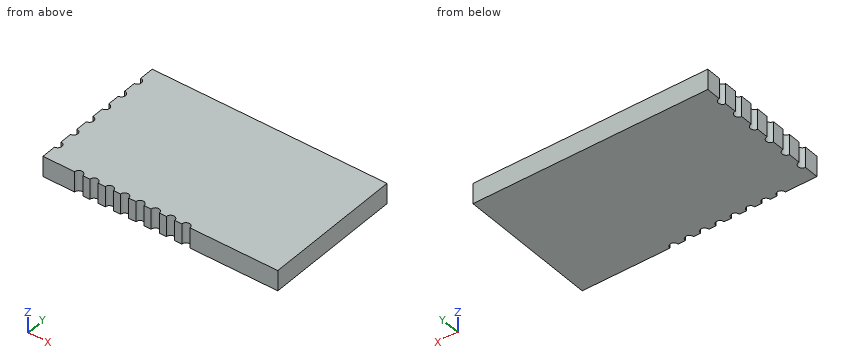
from build123d import *

# Parameters (mm, degrees)
EXTRUDE_1_DEPTH = 2


with BuildPart() as part:
    # Эскиз1 → Бобышка-Вытянуть1 (new body)
    with BuildSketch(Plane(origin=(0, 0, 0), x_dir=(-1, 0, 0), z_dir=(0, 0, -1))):
        with BuildLine():
            Line((-4.023063957, -1.975599526), (-3.323063957, -1.975599526))
            ThreePointArc((-3.323063957, -1.975599526), (-2.923063957, -1.575599526), (-2.523063957, -1.975599526))
            Line((-2.523063957, -1.975599526), (-1.823063957, -1.975599526))
            ThreePointArc((-1.823063957, -1.975599526), (-1.423063957, -1.575599526), (-1.023063957, -1.975599526))
            Line((-1.023063957, -1.975599526), (-0.323063957, -1.975599526))
            ThreePointArc((-0.323063957, -1.975599526), (0.076936043, -1.575599526), (0.476936043, -1.975599526))
            Line((0.476936043, -1.975599526), (1.176936043, -1.975599526))
            ThreePointArc((1.176936043, -1.975599526), (1.576936043, -1.575599526), (1.976936043, -1.975599526))
            Line((1.976936043, -1.975599526), (2.676936043, -1.975599526))
            ThreePointArc((2.676936043, -1.975599526), (3.076936043, -1.575599526), (3.476936043, -1.975599526))
            Line((3.476936043, -1.975599526), (4.176936043, -1.975599526))
            ThreePointArc((4.176936043, -1.975599526), (4.576936043, -1.575599526), (4.976936043, -1.975599526))
            Line((4.976936043, -1.975599526), (5.676936043, -1.975599526))
            ThreePointArc((5.676936043, -1.975599526), (6.076936043, -1.575599526), (6.476936043, -1.975599526))
            Line((6.476936043, -1.975599526), (9.576936043, -1.975599526))
            Line((9.576936043, -1.975599526), (9.576936043, -0.525599526))
            ThreePointArc((9.576936043, -0.525599526), (9.176936043, -0.125599526), (9.576936043, 0.274400474))
            Line((9.576936043, 0.274400474), (9.576936043, 1.474400474))
            ThreePointArc((9.576936043, 1.474400474), (9.176936043, 1.874400474), (9.576936043, 2.274400474))
            Line((9.576936043, 2.274400474), (9.576936043, 3.474400474))
            ThreePointArc((9.576936043, 3.474400474), (9.176936043, 3.874400474), (9.576936043, 4.274400474))
            Line((9.576936043, 4.274400474), (9.576936043, 5.474400474))
            ThreePointArc((9.576936043, 5.474400474), (9.176936043, 5.874400474), (9.576936043, 6.274400474))
            Line((9.576936043, 6.274400474), (9.576936043, 7.474400474))
            ThreePointArc((9.576936043, 7.474400474), (9.176936043, 7.874400474), (9.576936043, 8.274400474))
            Line((9.576936043, 8.274400474), (9.576936043, 9.474400474))
            ThreePointArc((9.576936043, 9.474400474), (9.176936043, 9.874400474), (9.576936043, 10.274400474))
            Line((9.576936043, 10.274400474), (9.576936043, 11.724400474))
            Line((9.576936043, 11.724400474), (-13.423063957, 11.724400474))
            Line((-13.423063957, 11.724400474), (-13.423063957, -1.975599526))
            Line((-13.423063957, -1.975599526), (-4.823063957, -1.975599526))
            ThreePointArc((-4.823063957, -1.975599526), (-4.423063957, -1.575599526), (-4.023063957, -1.975599526))
        make_face()
    extrude(amount=EXTRUDE_1_DEPTH)


solid = part.part
For this review, take the finished solid that the model builds, in its own axes (mm). Coordinates: 2 decimals unless noted, no trailing zeros. Write each loop counter-clockwise with the first axis right and the second up, starting at its lowest first coordinate (ties: lowest second). Pieces come first, ordered by that corner, then holes. Notation, with made-up numbers: (82, 61) -> (125, 61) arc R24 cw to (125, 92) -> close; hole circle Ø4 at (-17.75, 62.5). An arc over 180 degrees is marked (long way). Write each question's results on one line, items separated by ' | '. Start each with the question number.
1) Consider section A-A (y = 2). Write out the cut boundary in (x, z), plus the area to 3 significant figures.
2) Wall thickness on L1, parallel to X at y = 9.75, z = -0.7; L2, parallel to Y at x = -6.25, z = -0.75; L3, parallel to Y at x = -5.75, z = -1.4: over which ranges is each line inside the solid? List them lowest first. Write a range as [from, to].
3) Consider section B-B (x = 4.5). Write out the cut boundary in (y, z), plus the area to 3 significant figures.
Geometry says:
1) outline: (-9.2, -2) -> (13.42, -2) -> (13.42, 0) -> (-9.2, 0) -> close | area: 45.2 mm^2
2) L1: [-9.2, 13.42] | L2: [-1.61, 11.72] | L3: [-1.75, 11.72]
3) outline: (-1.58, -2) -> (11.72, -2) -> (11.72, 0) -> (-1.58, 0) -> close | area: 26.6 mm^2
